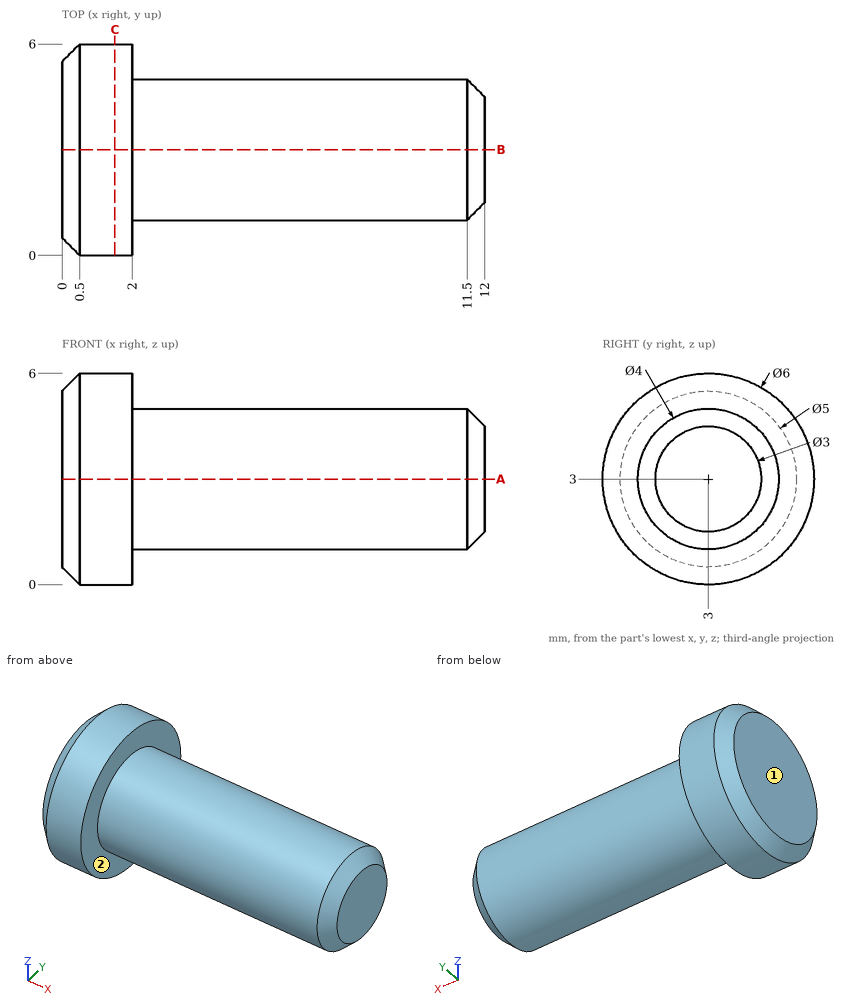
Source: three-view drawing plus pictorial views. Frame: mm from the lowest corner of the part. A direction names the side the tool comes from. Coordinates: 2 decimals unless noted, no trailing zeros. Order: outer loops, then holes, each group sorted by start corner. A loop starts at its lowest first (then second) coordinate and runs counter-clockwise, first axis right, second up.
Item 1: First-contact query: P1, Ø2, axis at x = 5, z = 1.5, coming from the -Y side. Flat tip, straight axial feed; report the tip coordinate or a pass-through.
Output values:
P1: stops at y = 1.06
Item 2: Cut plane C-C (x = 1.5). Return loops of the section in (y, z), plus the area to 3 significant figures.
Output values:
outline: circle Ø6 at (3, 3)
area: 28.3 mm2
Item 3: Cut plane A-A (z = 3). Return loops of the section in (x, y).
Output values:
outline: (0, 0.5) - (0.5, 0) - (2, 0) - (2, 1) - (11.5, 1) - (12, 1.5) - (12, 4.5) - (11.5, 5) - (2, 5) - (2, 6) - (0.5, 6) - (0, 5.5) - close
Item 4: Material intervals for line 1 (X direction, y = 4.55, z = 1.7); line 2 (X direction, y = 1.35, z = 4); line 3 (Z direction, x = 8.25, y = 1.9), sorted ascending.
Output values:
line 1: x = 0 to 2
line 2: x = 0 to 11.57
line 3: z = 1.33 to 4.67
Item 5: Set-up query: the marked faces 1 and 2. Return all of +Z, -Z, +X, -X, +Y, -Y with unobstructed straight access to the full face (end or side cutting, diameter ignored); none if empty.
Output values:
face 1: +Z, -Z, -X, +Y, -Y
face 2: +X
